from build123d import *

# Parameters (mm, degrees)
EXTRUDE_1_DEPTH = 15


with BuildPart() as part:
    # Эскиз1 → Повернуть1 (revolve)
    with BuildSketch(Plane(origin=(0, 0, 0), x_dir=(0, 0, -1), z_dir=(1, 0, 0))):
        Polygon((-176.350852961, 0), (40, 0), (40, 10), (-170.577350269, 10), align=None)
    revolve(axis=Axis((0, 0, 756.580802456), (0, 0, -1)))

    # Эскиз4 → Бобышка-Вытянуть1 (add)
    with BuildSketch(Plane(origin=(0, 0, -40), x_dir=(-1, 0, 0), z_dir=(0, 0, -1))):
        Polygon((0, 8.660254038), (-7.5, 4.330127019), (-7.5, -4.330127019), (0, -8.660254038), (7.5, -4.330127019), (7.5, 4.330127019), align=None)
    extrude(amount=EXTRUDE_1_DEPTH)


solid = part.part
Part model, mm, in its own coordinate system. A direction names the side the tool comes from. Round coordinates to 2 decimals unless told otherwise and drop trailing zeros. Loops run counter-clockwise (first coordinate to the right, second up) from the corner with the lowest first, then second, coordinate; pieces in that order, holes last. Notation, with made-up numbers: (-29, 69.5) - (7, 69.5) arc R18 ccw to (7, 103.5) - close; hole circle Ø4 at (34, -17). An arc over 180 degrees is marked (long way). Answer as a JSON object with one key per item and string values.
Item 1: Band-saw the part on A-A on z = 9.5. List the corners of the cut face in (x, y), plus the area to 3 significant figures.
Output:
{"outline": "circle Ø20 at (0, 0)", "area": "314 mm2"}
Item 2: Pin check, flat tips, straight feed: pin 1 (10 mm diameter, centred on y = 3, z = 116, fed in from +X); pin 2 (1 mm diameter, centred on x = 7, z = 44.5, fed in from -Y); pin 3 (4.5 mm diameter, centred on y = 1.5, z = -48, fed in from -X); pin 4 (9.5 mm diameter, centred on y = 0, z = -48.5, fed in from +X). Stop position of each tip, or through.
Output:
{"pin 1": "x = 10", "pin 2": "y = -7.6", "pin 3": "x = -7.5", "pin 4": "x = 7.5"}
Item 3: Tool access for faces 1 (the face through (-7.5, 0, -47)), 2 (the face through (-3.698, -6.526, -47.395)), 3 (the face through (7.5, 0, -47)), 4 (the face through (-3.802, 6.465, -47.395)), 5 (the face through (3.802, -6.465, -47.395)): list every direction of +Z, -Z, +X, -X, +Y, -Y with a clear straight run to the whole face (end or side of a thin tool).
Output:
{"face 1": "-Z, -X, +Y, -Y", "face 2": "-Z, -X, -Y", "face 3": "-Z, +X, +Y, -Y", "face 4": "-Z, -X, +Y", "face 5": "-Z, +X, -Y"}
Item 4: Wall check: L1, parallel to Y at x = 0.25, z = 161.5; L2, parallel to X at y = -9, z = 24; L3, parallel to Z at x = 4.25, y = -5.25. Give the ranges that are in metal, low to high.
Output:
{"L1": "-10 to 10", "L2": "-4.36 to 4.36", "L3": "-55 to 172.45"}
